from build123d import *

# Parameters (mm, degrees)
ESQUISSE1_W             = 160
ESQUISSE1_H             = 90
EXTRUSION1_DEPTH        = 50
CONG_1_R                = 25
CONG_2_R                = 15
COQUE1_T                = -3
ESQUISSE2_W             = 50
ESQUISSE2_H             = 15
ENL_V_MAT_EXTRU_1_DEPTH = 2
CONG_4_R                = 2
CONG_5_R                = 2
CONG_6_R                = 2
CONG_7_R                = 2
CONG_4_OF_SYM_TRIE1_R   = 2
CONG_5_OF_SYM_TRIE1_R   = 2
CONG_6_OF_SYM_TRIE1_R   = 2
CONG_7_OF_SYM_TRIE1_R   = 2


with BuildPart() as part:
    # Esquisse1 → Extrusion1 (new body)
    with BuildSketch(Plane(origin=(0, 0, 0), x_dir=(1, 0, 0), z_dir=(0, 1, 0))):
        with Locations((35.341232877, 23.705753425)):
            Rectangle(ESQUISSE1_W, ESQUISSE1_H)
    extrude(amount=EXTRUSION1_DEPTH)

    # Congé1
    cong_1_edges = [part.edges().sort_by_distance(p)[0] for p in [
        (115.341232877, 50, -23.705753425),
        (-44.658767123, 50, -23.705753425),
    ]]
    fillet(cong_1_edges, radius=CONG_1_R)

    # Congé2
    cong_2_edges = [part.edges().sort_by_distance(p)[0] for p in [
        (35.341232877, 50, 21.294246575),
        (35.341232877, 50, -68.705753425),
        (115.341232877, 12.5, 21.294246575),
        (-44.658767123, 12.5, 21.294246575),
        (108.018902406, 42.67766953, 21.294246575),
        (-37.336436653, 42.67766953, 21.294246575),
        (-44.658767123, 12.5, -68.705753425),
        (115.341232877, 12.5, -68.705753425),
        (108.018902406, 42.67766953, -68.705753425),
        (-37.336436653, 42.67766953, -68.705753425),
    ]]
    fillet(cong_2_edges, radius=CONG_2_R)

    # Coque1
    coque1_openings = [part.faces().sort_by_distance(p)[0] for p in [
        (35.341232877, 0, -23.705753425),
    ]]
    offset(amount=COQUE1_T, openings=coque1_openings, kind=Kind.INTERSECTION)

    # Esquisse2 → Enlèv. mat.-Extru.1 (cut)
    with BuildSketch(Plane.XY.offset(21.294246575)):
        with Locations((35.341232877, 22.5)):
            Rectangle(ESQUISSE2_W, ESQUISSE2_H)
    enl_v_mat_extru_1 = extrude(amount=-ENL_V_MAT_EXTRU_1_DEPTH, mode=Mode.SUBTRACT)

    # Congé4
    cong_4_edges = [part.edges().sort_by_distance(p)[0] for p in [
        (35.341232877, 15, 19.294246575),
    ]]
    fillet(cong_4_edges, radius=CONG_4_R - 0.0001)  # a hair under: the kernel refuses the full size

    # Congé5
    cong_5_edges = [part.edges().sort_by_distance(p)[0] for p in [
        (35.341232877, 30, 19.294246575),
    ]]
    fillet(cong_5_edges, radius=CONG_5_R - 0.0001)  # a hair under: the kernel refuses the full size

    # Congé6
    cong_6_edges = [part.edges().sort_by_distance(p)[0] for p in [
        (10.341232877, 15.585757148, 19.880003724),
        (10.341232877, 22.5, 19.294246575),
        (10.341232877, 29.414242852, 19.880003724),
    ]]
    fillet(cong_6_edges, radius=CONG_6_R - 0.0001)  # a hair under: the kernel refuses the full size

    # Congé7
    cong_7_edges = [part.edges().sort_by_distance(p)[0] for p in [
        (60.341232877, 22.5, 19.294246575),
        (60.341232877, 15.585757148, 19.880003724),
        (60.341232877, 29.414242852, 19.880003724),
    ]]
    fillet(cong_7_edges, radius=CONG_7_R - 0.0001)  # a hair under: the kernel refuses the full size

    # Symétrie1: Enlèv. mat.-Extru.1 across plane
    add(enl_v_mat_extru_1.mirror(Plane.XY.offset(-23.705753425)), mode=Mode.SUBTRACT)

    # Congé4 of Symétrie1
    cong_4_of_sym_trie1_edges = [part.edges().sort_by_distance(p)[0] for p in [
        (35.341232877, 15, -66.705753425),
    ]]
    fillet(cong_4_of_sym_trie1_edges, radius=CONG_4_OF_SYM_TRIE1_R - 0.0001)  # a hair under: the kernel refuses the full size

    # Congé5 of Symétrie1
    cong_5_of_sym_trie1_edges = [part.edges().sort_by_distance(p)[0] for p in [
        (35.341232877, 30, -66.705753425),
    ]]
    fillet(cong_5_of_sym_trie1_edges, radius=CONG_5_OF_SYM_TRIE1_R - 0.0001)  # a hair under: the kernel refuses the full size

    # Congé6 of Symétrie1
    cong_6_of_sym_trie1_edges = [part.edges().sort_by_distance(p)[0] for p in [
        (10.341232877, 15.585757148, -67.291510573),
        (10.341232877, 22.5, -66.705753425),
        (10.341232877, 29.414242852, -67.291510573),
    ]]
    fillet(cong_6_of_sym_trie1_edges, radius=CONG_6_OF_SYM_TRIE1_R - 0.0001)  # a hair under: the kernel refuses the full size

    # Congé7 of Symétrie1
    cong_7_of_sym_trie1_edges = [part.edges().sort_by_distance(p)[0] for p in [
        (60.341232877, 22.5, -66.705753425),
        (60.341232877, 15.585757148, -67.291510573),
        (60.341232877, 29.414242852, -67.291510573),
    ]]
    fillet(cong_7_of_sym_trie1_edges, radius=CONG_7_OF_SYM_TRIE1_R - 0.0001)  # a hair under: the kernel refuses the full size


solid = part.part
Could you check a few things on this model? Use its own coordinates, in mm. A direction names the side the tool comes from. Give positions to 0.01 mm unless a question says otherwise; leave off trailing zeros. Order: outer loops, then holes, each group sorted by start corner. A loop starts at its lowest first (then second) coordinate and runs counter-clockwise, first axis right, second up.
Item 1: If we section it at A-A, the plane z = 3: Write out the boundary of the cut face in (x, y).
Item 2: I need wall thicknesses on line 1 (X direction, y = 5, z = -15); line 2 (Z direction, x = 91.5, y = 10.5); line 3 (Y direction, x = 74.5, z = -29). Which ranges of each line are inside material? Lowest first, please.
Item 3: For faces 1 (the face through (35, 23, -66.706)), 2 (the face through (34, 17, -65.706)), 3 (the face through (-37.53, 42.48, -24.13)), which set-ups out of +Z, -Z, +X, -X, +Y, -Y let a thin tool reach every point of the face, with its end or its side?
Item 4: If we mould it in two halves opening along Z, with no side actions, what happens to faces 4 (the face through (110.83, 12.33, -64.43)), 5 (the face through (115.341, 12, -23)), 6 (the face through (34, 17, 18.294))? For each: pulls with the +Z half, pulls with the -Z half, needs draft (parallel to the pull), parting line crosses it, or undercut.
Item 5: If we section it at C-C, the plane y = 10: Write out the boundary of the cut face in (x, z), plus the area to 3 significant figures.
Item 6: I'm going to push flat-ended pins straight in: pin 1 (4 mm diameter, centred on x = -8.5, z = -56, fed in from -Y); pin 2 (1 mm diameter, centred on x = 30.5, y = 41, fed in from -Z); pin 3 (12 mm diameter, centred on x = 13.5, z = -2, fed in from -Y). Where does each tip first touch, or does it pass through?
Item 7: If we section it at B-B, the plane x = 7: Write out the boundary of the cut face in (y, z), plus the area to 3 significant figures.
Values:
1. outline: (-44.66, 0) - (-41.66, 0) - (-41.66, 25) arc R22 cw to (-19.66, 47) - (90.34, 47) arc R22 cw to (112.34, 25) - (112.34, 0) - (115.34, 0) - (115.34, 25) arc R25 ccw to (90.34, 50) - (-19.66, 50) arc R25 ccw to (-44.66, 25) - close
2. line 1: x = -44.66 to -41.66, 112.34 to 115.34
2. line 2: z = -68.71 to -65.71, 18.29 to 21.29
2. line 3: y = 47 to 50
3. face 1: -Z
3. face 2: -Y
3. face 3: +Z, -Z, -X, +Y
4. face 4: pulls with the -Z half
4. face 5: needs draft
4. face 6: undercut
5. outline: (-44.66, -53.71) arc R15 ccw to (-29.66, -68.71) - (100.34, -68.71) arc R15 ccw to (115.34, -53.71) - (115.34, 6.29) arc R15 ccw to (100.34, 21.29) - (-29.66, 21.29) arc R15 ccw to (-44.66, 6.29) - close; hole (-41.66, -53.71) arc R12 ccw to (-29.66, -65.71) - (100.34, -65.71) arc R12 ccw to (112.34, -53.71) - (112.34, 6.29) arc R12 ccw to (100.34, 18.29) - (-29.66, 18.29) arc R12 ccw to (-41.66, 6.29) - close
5. area: 1,390 mm2
6. pin 1: stops at y = 46.21
6. pin 2: stops at z = -67.66
6. pin 3: stops at y = 47
7. outline: (0, -68.71) - (35, -68.71) arc R15 ccw to (50, -53.71) - (50, 6.29) arc R15 ccw to (35, 21.29) - (0, 21.29) - (0, 18.29) - (35, 18.29) arc R12 cw to (47, 6.29) - (47, -53.71) arc R12 cw to (35, -65.71) - (0, -65.71) - close
7. area: 517 mm2
